CAD build for the part. Positions are in the model's coordinates, mm. Round coordinates to 2 decimals unless told otherwise and drop trailing zeros. Write each loop counter-clockwise with the first axis right and the second up, starting at its lowest first coordinate (ties: lowest second). Pieces come first, ordered by that corner, then holes. Notation, with made-up numbers: (22.25, 76.25) - (77.25, 76.25) arc R34 ccw to (77.25, 110.25) - close; hole circle Ø9 at (63, 30.5). An arc over 180 degrees is marked (long way). Answer in a Markdown table with one row per item.
```python
from build123d import *

# Parameters (mm, degrees)
SKETCH1_R               = 4.7625
BOSS_EXTRUDE1_DEPTH     = 285.75
CUT_EXTRUDE1_DEPTH      = 5.7625
CUT_EXTRUDE1_DEPTH_BACK = 5.7625
F_8_32_TAPPED_HOLE1_D   = 3.4544


with BuildPart() as part:
    # Sketch1 → Boss-Extrude1 (new body)
    with BuildSketch(Plane(origin=(0, 0, 0), x_dir=(1, 0, 0), z_dir=(0, 1, 0))):
        Circle(SKETCH1_R)
    extrude(amount=BOSS_EXTRUDE1_DEPTH)

    # Sketch2 → Cut-Extrude1 (cut, two sides)
    with BuildSketch(Plane.XY) as cut_extrude1_sk:
        with BuildLine():
            Line((-1.5875, -50.8), (-1.5875, 50.8))
            ThreePointArc((-1.5875, 50.8), (0, 52.3875), (1.5875, 50.8))
            Line((1.5875, 50.8), (1.5875, -50.8))
            ThreePointArc((1.5875, -50.8), (0, -52.3875), (-1.5875, -50.8))
        make_face()
    extrude(amount=CUT_EXTRUDE1_DEPTH, mode=Mode.SUBTRACT)
    extrude(cut_extrude1_sk.sketch, amount=-CUT_EXTRUDE1_DEPTH_BACK, mode=Mode.SUBTRACT)

    # #8-32 Tapped Hole1 (through all)
    with Locations(Plane(origin=(0, 0, -4.7625), x_dir=(-1, 0, 0), z_dir=(0, 0, -1))):
        with Locations((0, 279.4)):
            Hole(F_8_32_TAPPED_HOLE1_D / 2)


solid = part.part
```
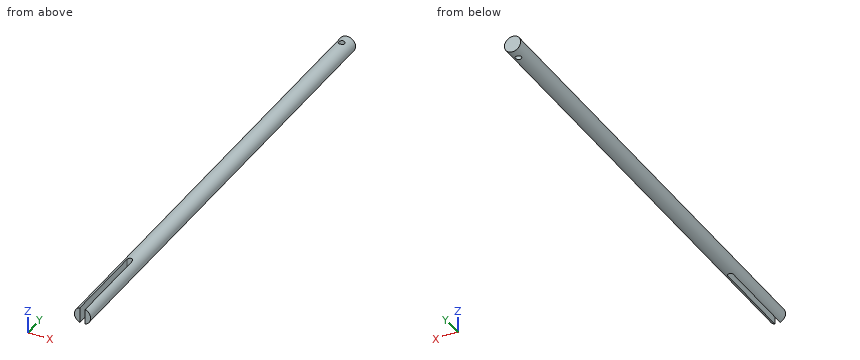
Q1. Saw through at A-A on x = 0. List the corners of the cut face in (y, z), then the cut area to 3 significant figures.
Computed:
| item | result |
|---|---|
| outline | (52.39, -4.76) - (277.67, -4.76) - (277.67, 4.76) - (52.39, 4.76) - close; (281.13, -4.76) - (285.75, -4.76) - (285.75, 4.76) - (281.13, 4.76) - close |
| area | 2,190 mm2 |
Q2. Flat gauge pins, fed straight in: pin 1 (2 mm diameter, centred on y = 152, z = -3, fed in from +X); pin 2 (4 mm diameter, centred on y = 188, z = 3.5, fed in from -X); pin 3 (2 mm diameter, centred on y = 117.5, z = 3, fed in from -X). Where does each tip first touch, or does it go through?
Computed:
| item | result |
|---|---|
| pin 1 | stops at x = 4.32 |
| pin 2 | stops at x = -4.52 |
| pin 3 | stops at x = -4.32 |
Q3. Drill centre lines: line 1 (Y direction, x = 0, z = 3.5); line 2 (X direction, y = 279.4, z = 0); line 3 (Z direction, x = 0.25, y = 263). Where is each one in solid material? Low to high.
Computed:
| item | result |
|---|---|
| line 1 | y = 52.39 to 277.67, 281.13 to 285.75 |
| line 2 | x = -4.76 to -1.73, 1.73 to 4.76 |
| line 3 | z = -4.76 to 4.76 |
Q4. Saw through at C-C on y = 64.5. List the corners of the cut face in (x, z) (1 decimal), then the cut area to 3 significant figures.
Computed:
| item | result |
|---|---|
| outline | circle Ø9.5 at (0, 0) |
| area | 71.3 mm2 |
